from build123d import *

# Parameters (mm, degrees)
F2_W     = 38.1
F2_H     = 38.1
F3_DEPTH = 38.1
F4_W     = 38.1
F4_H     = 38.1
F5_DEPTH = 38.1
F6_DEPTH = 38.1


with BuildPart() as f1:
    # F0 (on Front) → F1 (revolve)
    with BuildSketch(Plane.XZ):
        with BuildLine():
            ThreePointArc((-38.412295, -29.251639), (-19.228771, -10.201639), (-38.412295, 8.848361))
            Line((-38.412295, 8.848361), (-38.412295, -29.251639))
        make_face()
    revolve(axis=Axis((-38.412295, 0, -10.201639), (0, 0, -1)))

    # F2 (on Top) → F3 (join)
    with BuildSketch(Plane.XY):
        with Locations((-39.272306, 0)):
            Rectangle(F2_W, F2_H)
    extrude(amount=F3_DEPTH)

    # F4 (on Top) → F5 (join)
    with BuildSketch(Plane.XY):
        with Locations((-38.76623, 0.147158)):
            Rectangle(F4_W, F4_H)
    extrude(amount=F5_DEPTH)

    # F5_face (on face) → F6 (join)
    with BuildSketch(Plane(origin=(-39.019268, 0.073579, 38.1), x_dir=(1, 0, 0), z_dir=(0, 0, 1))):
        Polygon((19.303038, 19.123579), (-18.796962, 19.123579), (-18.796962, 18.976421), (-19.303038, 18.976421), (-19.303038, -19.123579), (18.796962, -19.123579), (18.796962, -18.976421), (19.303038, -18.976421), align=None)
    extrude(amount=F6_DEPTH)


solid = f1.part
Could you check a few things on this model? Use its own coordinates, in mm. Coordinates: 2 decimals unless noted, no trailing zeros. Write each loop counter-clockwise with the first axis right and the second up, starting at its lowest first coordinate (ties: lowest second). Pieces come first, ordered by that corner, then holes. Notation, with made-up numbers: (3, 56.25) - (32, 56.25) arc R23 ccw to (32, 82.25) - close; hole circle Ø8 at (69, -36). An arc over 180 degrees is marked (long way). Put each result on its own line as item: value. Start each with the question number.
Q1. I'm going to push flat-ended pins straight in: P1, Ø19, axis at x = -34, y = 5, coming from the -Z side; P2, Ø11.5, axis at x = -43, z = 32, coming from the -Y side; P3, Ø19, axis at y = 0, z = 33.5, coming from the +X side; P4, Ø2, axis at x = -35, y = -8, coming from the -Z side. Where does each tip first touch, or does it pass through?
Q2. Thinking about a two-plate mould opening in Z: for faces 1 (the flat face through (-19.716, 0, 38)), 2 (the flat face through (-39, 17, 0)), 3 (the flat face through (-39, 0, 76.2)), which applies, pulls with the +Z half, pulls with the -Z half, needs draft (parallel to the pull), parting line crosses it, or undercut?
Q3. Please list where these lines run through material, in increasing order: L1, parallel to X at y = -6.5, z = 22.5; L2, parallel to Y at x = -23, z = 29.5; L3, parallel to Z at x = -51, y = -12.
Q4. I want a section at A-A on z = 18.5. Write out the boundary of the cut face in (x, y), plus the area to 3 significant figures.
Checks:
1. P1: z = -29.25
1. P2: y = -19.05
1. P3: x = -19.72
1. P4: z = -27.69
2. face 1: needs draft
2. face 2: undercut
2. face 3: pulls with the +Z half
3. L1: -58.32 to -19.72
3. L2: -19.05 to 19.2
3. L3: -18.27 to -2.13, 0 to 76.2
4. outline: (-58.32, -19.05) - (-20.22, -19.05) - (-20.22, -18.9) - (-19.72, -18.9) - (-19.72, 19.2) - (-57.82, 19.2) - (-57.82, 19.05) - (-58.32, 19.05) - close
4. area: 1,480 mm²
